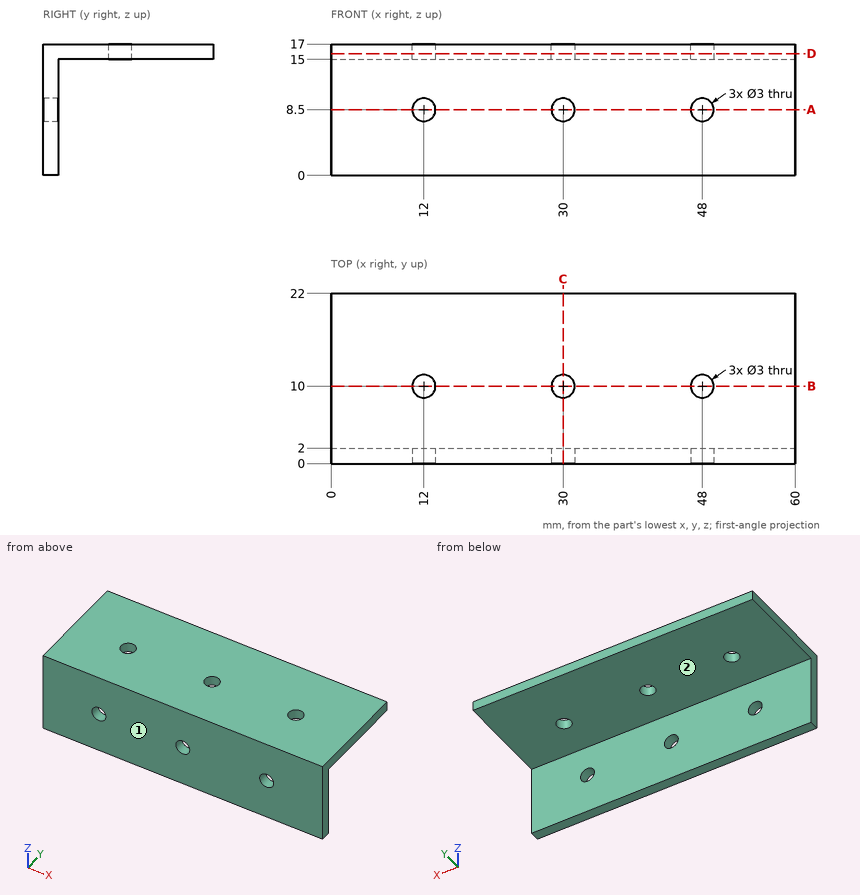
Could you check a few things on this drawing? It's one solid part, dimensions in mm from its lowest x, y, z. A direction names the side the tool comes from. Give positions to 0.01 mm unless a question says otherwise; leave off trailing zeros. Loops run counter-clockwise (first coordinate to the right, second up) from the corner with the lowest first, then second, coordinate; pieces in that order, holes last. Notation, with made-up numbers: (3, 55.5) -> (34, 55.5) arc R10 ccw to (34, 67.5) -> close; hole circle Ø11 at (50.5, 31.5). An arc over 180 degrees is marked (long way). Use one line per item in the form item = value. Start each with the question number.
1) Imagine slicing it at A-A (z = 8.5). Please give me the cut outline in (x, y).
2) Please list where these lines run through material, in increasing order: line 1 along X through (y, z) = (0.5, 8.5); line 2 along Y through (x, z) = (12, 16.1); line 3 along Y through (x, z) = (31.5, 9).
3) Which directions (+Z, -Z, +X, -X, +Y, -Y) give clear straight access to the entire face, cutting with the end or side of a thin tool? Please do the marked faces 1 and 2.
4) Imagine slicing it at B-B (y = 10). Please give me the cut outline in (x, z), then the cut area to 3 significant figures.
5) Imagine slicing it at D-D (z = 15.75). Please give me the cut outline in (x, y).
6) For P1, Ø3.5, axis at x = 30, z = 8.5, coming from the +Y side; P2, Ø8, axis at x = 38, y = 13.5, coming from the -Z side, each with a flat end and sliding along its axis, tell me the tip position at first contact or that it passes through.
7) Imagine slicing it at C-C (x = 30). Please give me the cut outline in (y, z), then the cut area to 3 significant figures.
Check values:
q1.outline = (0, 0) -> (10.5, 0) -> (10.5, 2) -> (0, 2) -> close; (13.5, 0) -> (28.5, 0) -> (28.5, 2) -> (13.5, 2) -> close; (31.5, 0) -> (46.5, 0) -> (46.5, 2) -> (31.5, 2) -> close; (49.5, 0) -> (60, 0) -> (60, 2) -> (49.5, 2) -> close
q2.line_1 = 0 to 10.5, 13.5 to 28.5, 31.5 to 46.5, 49.5 to 60
q2.line_2 = 0 to 8.5, 11.5 to 22
q2.line_3 = 0 to 2
q3.face_1 = +Z, -Z, +X, -X, -Y
q3.face_2 = -Z, +X, -X, +Y
q4.outline = (0, 15) -> (10.5, 15) -> (10.5, 17) -> (0, 17) -> close; (13.5, 15) -> (28.5, 15) -> (28.5, 17) -> (13.5, 17) -> close; (31.5, 15) -> (46.5, 15) -> (46.5, 17) -> (31.5, 17) -> close; (49.5, 15) -> (60, 15) -> (60, 17) -> (49.5, 17) -> close
q4.area = 102 mm^2
q5.outline = (0, 0) -> (60, 0) -> (60, 22) -> (0, 22) -> close; hole circle Ø3 at (12, 10); hole circle Ø3 at (30, 10); hole circle Ø3 at (48, 10)
q6.P1 = 2
q6.P2 = 15
q7.outline = (0, 0) -> (2, 0) -> (2, 7) -> (0, 7) -> close; (0, 10) -> (2, 10) -> (2, 15) -> (8.5, 15) -> (8.5, 17) -> (0, 17) -> close; (11.5, 15) -> (22, 15) -> (22, 17) -> (11.5, 17) -> close
q7.area = 62.0 mm^2
